from build123d import *

# Parameters (mm, degrees)
BOSS_EXTRUDE1_DEPTH     = 115
CUT_EXTRUDE4_DEPTH      = 56
CUT_EXTRUDE4_DEPTH_BACK = 156
FILLET1_R               = 20
SKETCH4_R               = 15
CUT_EXTRUDE5_DEPTH      = 56
CUT_EXTRUDE5_DEPTH_BACK = 148


with BuildPart() as part:
    # Sketch1 → Boss-Extrude1 (new body)
    with BuildSketch(Plane(origin=(0, 0, 0), x_dir=(0, 0, -1), z_dir=(1, 0, 0))):
        with BuildLine():
            Line((0, 0), (210, 0))
            Line((210, 0), (210, 30))
            Line((210, 30), (155, 30))
            Line((155, 30), (155, 172.5))
            Line((155, 172.5), (163, 172.5))
            Line((163, 172.5), (163, 217.5))
            Line((163, 217.5), (155, 217.5))
            Line((155, 217.5), (155, 310))
            Line((155, 310), (55, 310))
            Line((55, 310), (55, 235))
            Line((55, 235), (115, 235))
            ThreePointArc((115, 235), (155, 195), (115, 155))
            Line((115, 155), (55, 155))
            Line((55, 155), (55, 30))
            Line((55, 30), (0, 30))
            Line((0, 30), (0, 0))
        make_face()
    extrude(amount=BOSS_EXTRUDE1_DEPTH)

    # Sketch2 → Cut-Extrude4 (cut, two sides)
    with BuildSketch(Plane(origin=(0, 0, -155), x_dir=(-1, 0, 0), z_dir=(0, 0, -1))) as cut_extrude4_sk:
        with BuildLine():
            Line((0, 172.5), (-17.5, 172.5))
            Line((-17.5, 172.5), (-17.5, 80))
            Line((-17.5, 80), (-22.5, 80))
            ThreePointArc((-22.5, 80), (-26.035533906, 78.535533906), (-27.5, 75))
            Line((-27.5, 75), (-27.5, 50))
            ThreePointArc((-27.5, 50), (-21.642135624, 35.857864376), (-7.5, 30))
            Line((-7.5, 30), (0, 30))
            Line((0, 30), (0, 172.5))
        make_face()
        with BuildLine():
            Line((-97.5, 172.5), (-97.5, 302.819293264))
            ThreePointArc((-97.5, 302.819293264), (-77.819710562, 308.190588667), (-57.5, 310))
            Line((-57.5, 310), (-115, 310))
            Line((-115, 310), (-115, 172.5))
            Line((-115, 172.5), (-97.5, 172.5))
        make_face()
        with BuildLine():
            Line((-97.5, 80), (-97.5, 172.5))
            Line((-97.5, 172.5), (-115, 172.5))
            Line((-115, 172.5), (-115, 30))
            Line((-115, 30), (-107.5, 30))
            ThreePointArc((-107.5, 30), (-93.357864376, 35.857864376), (-87.5, 50))
            Line((-87.5, 50), (-87.5, 75))
            ThreePointArc((-87.5, 75), (-88.964466094, 78.535533906), (-92.5, 80))
            Line((-92.5, 80), (-97.5, 80))
        make_face()
        with BuildLine():
            Line((0, 310), (-57.5, 310))
            ThreePointArc((-57.5, 310), (-37.180289438, 308.190588667), (-17.5, 302.819293264))
            Line((-17.5, 302.819293264), (-17.5, 172.5))
            Line((-17.5, 172.5), (0, 172.5))
            Line((0, 172.5), (0, 310))
        make_face()
    extrude(amount=CUT_EXTRUDE4_DEPTH, mode=Mode.SUBTRACT)
    extrude(cut_extrude4_sk.sketch, amount=-CUT_EXTRUDE4_DEPTH_BACK, mode=Mode.SUBTRACT)

    # Fillet1
    fillet1_edges = [part.edges().sort_by_distance(p)[0] for p in [
        (57.5, 30, -155),
        (57.5, 30, -55),
    ]]
    fillet(fillet1_edges, radius=FILLET1_R)

    # Sketch4 → Cut-Extrude5 (cut, two sides)
    with BuildSketch(Plane(origin=(0, 0, -155), x_dir=(-1, 0, 0), z_dir=(0, 0, -1))) as cut_extrude5_sk:
        with Locations((-57.5, 120)):
            Circle(SKETCH4_R)
        with Locations((-57.5, 270)):
            Circle(SKETCH4_R)
    extrude(amount=CUT_EXTRUDE5_DEPTH, mode=Mode.SUBTRACT)
    extrude(cut_extrude5_sk.sketch, amount=-CUT_EXTRUDE5_DEPTH_BACK, mode=Mode.SUBTRACT)


solid = part.part
The model under review builds one solid part; all positions refer to its coordinate system, in mm. A direction names the side the tool comes from. Round coordinates to 2 decimals unless told otherwise and drop trailing zeros. Loops run counter-clockwise (first coordinate to the right, second up) from the corner with the lowest first, then second, coordinate; pieces in that order, holes last. Notation, with made-up numbers: M 48.25,-9 L 93.25,-9 A8 cw 93.25,2 Z; hole C -38.5,41.25 d2. An arc over 180 degrees is marked long. Answer as a JSON object with one key per item and string values.
Item 1: Tool access review of faces 4 (the face through (27.5, 63, -106)), 5 (the face through (6, 30, -130)), 6 (the face through (57, 155, -85)), 7 (the face through (57, 290, -55)), 8 (the face through (57, 253, -155)): name each direction out of +Z, -Z, +X, -X, +Y, -Y from which nothing blocks a thin tool from reaching the whole face with its end or side.
Check sheet entries:
{"face 4": "+Z, -Z, -X", "face 5": "+Y", "face 6": "+Z, +X, -X", "face 7": "+Z, +X, -X, +Y", "face 8": "-Z, +X, -X, +Y"}
Item 2: We need section D-D, the plane y = 264. State the section outline as (x, z) points.
Check sheet entries:
{"outline": "M 17.5,-155 L 43.75,-155 L 43.75,-55 L 17.5,-55 Z; M 71.25,-155 L 97.5,-155 L 97.5,-55 L 71.25,-55 Z"}
Item 3: Clearance check with flat-ended pins moving along their axes: P1, Ø4, axis at y = 258, z = -139, coming from the -X side; P2, Ø24, axis at x = 73, y = 83, coming from the +Z side; P3, Ø5.5, axis at x = 94, z = -88, coming from the -Y side; P4, Ø4, axis at x = 70.5, z = -160, coming from the +Y side. State where each tip first meets the part, or that it passes through.
Check sheet entries:
{"P1": "x = 17.5", "P2": "z = -55", "P3": "y = 0", "P4": "y = 217.5"}
Item 4: We need section C-C, the plane x = 66. State the section outline as (y, z) points, and give its area (3 significant figures).
Check sheet entries:
{"outline": "M 0,-210 L 30,-210 L 30,-175 A20 cw 50,-155 L 107.64,-155 L 107.64,-55 L 50,-55 A20 cw 30,-35 L 30,0 L 0,0 Z; M 132.36,-155 L 172.5,-155 L 172.5,-163 L 217.5,-163 L 217.5,-155 L 257.64,-155 L 257.64,-55 L 235,-55 L 235,-115 A40 cw 155,-115 L 155,-55 L 132.36,-55 Z; M 282.36,-155 L 309.69,-155 L 309.69,-55 L 282.36,-55 Z", "area": "22,500 mm2"}
Item 5: For line 1 along Y through (x, z) = (57.5, -96); line 2 along Y through (x, z) = (57, -133); line 3 along Y through (x, z) = (53, -188), list the stretches that pass through material, from the lowest coordinate up.
Check sheet entries:
{"line 1": "0 to 105, 135 to 155, 235 to 255, 285 to 310", "line 2": "0 to 105.01, 134.99 to 159.28, 230.72 to 255.01, 284.99 to 310", "line 3": "0 to 30"}
Item 6: We need section B-B, the plane y = 120. State the section outline as (x, z) points, and give its area (3 significant figures).
Check sheet entries:
{"outline": "M 17.5,-155 L 42.5,-155 L 42.5,-55 L 17.5,-55 Z; M 72.5,-155 L 97.5,-155 L 97.5,-55 L 72.5,-55 Z", "area": "5,000 mm2"}
Item 7: We need section A-A, the plane z = -111. State the section outline as (x, y) points.
Check sheet entries:
{"outline": "M 0,0 L 115,0 L 115,30 L 107.5,30 A20 cw 87.5,50 L 87.5,75 A5 cw 92.5,80 L 97.5,80 L 97.5,155 L 17.5,155 L 17.5,80 L 22.5,80 A5 cw 27.5,75 L 27.5,50 A20 cw 7.5,30 L 0,30 Z; M 17.5,235 L 97.5,235 L 97.5,302.82 A115 ccw 17.5,302.82 Z; hole C 57.5,120 d30; hole C 57.5,270 d30"}
Item 8: The part is to be moulded in two halves that separate along Y. For faces 1 (the face through (57, 172.5, -159)), 2 (the face through (57, 217.5, -159)), 3 (the face through (57, 195, -163)), say which applies: +Y half, -Y half, draft (parallel to the pull), parting line (faces both ways), or undercut.
Check sheet entries:
{"face 1": "undercut", "face 2": "+Y half", "face 3": "draft"}
